For this review, take the finished solid that the model builds, in its own axes (mm). Give positions to 0.01 mm unless a question says otherwise; leave off trailing zeros. Order: outer loops, then holes, each group sorted by start corner. A loop starts at its lowest first (then second) coordinate and runs counter-clockwise, first axis right, second up.
Autodesk Inventor part; units mm, degrees
ref_plane "YZ Plane" through (0, 0, 0) normal (1, 0, 0) x (0, 1, 0)
ref_plane "XZ Plane" through (0, 0, 0) normal (0, 1, 0) x (-1, 0, 0)
ref_plane "XY Plane" through (0, 0, 0) normal (0, 0, 1) x (1, 0, 0)
ref_plane "Work Plane1" through (0, 0, 0) normal (0, 0, 1) x (1, 0, 0)
sketch "Sketch1" plane through (0, 0, 0) normal (0, 0, 1) x (1, 0, 0)
  line L0 (60, 154.3122) -> (60, -124.8582) construction
  line L1 (-40, -55.6878) -> (-40, 204.3122)
  line L2 (-40, 204.3122) -> (160, 204.3122)
  line L3 (160, 204.3122) -> (160, -55.6878)
  arc A0 (-2.8578, 10.3642) -> (-5.2959, -9.3561) centre (-2.949, 0.3646) ccw
  arc A1 (20.3319, 92.7038) -> (13.1645, 74.1711) centre (17.8081, 83.0275) ccw
  arc A2 (68.5267, 149.0877) -> (51.4733, 149.0877) centre (60, 154.3122) ccw
  arc A3 (106.8355, 74.1711) -> (99.6681, 92.7038) centre (102.1919, 83.0275) ccw
  arc A4 (125.2959, -9.3561) -> (122.8578, 10.3642) centre (122.949, 0.3646) ccw
  line L4 (-3, -12.2723) -> (-3, -52.6878)
  line L5 (0.0792, 12.6334) -> (14.681, 70.7835)
  line L6 (23.7332, 94.1894) -> (51.5594, 146.1031)
  line L7 (68.4406, 146.1031) -> (96.2668, 94.1894)
  line L8 (105.319, 70.7835) -> (119.9208, 12.6334)
  line L9 (123, -12.2723) -> (123, -52.6878)
  line L10 (160, -55.6878) -> (126, -55.6878)
  line L11 (-6, -55.6878) -> (-40, -55.6878)
  line L12 (-3, -0.4636) -> (-3, -80.75)
  line L13 (17.557, 82.2366) -> (-2.7968, 1.1803)
  line L14 (54.0507, 150.7511) -> (18.1545, 83.7816)
  line L15 (101.8455, 83.7816) -> (65.9493, 150.7511)
  line L16 (122.7968, 1.1803) -> (102.443, 82.2366)
  line L17 (123, -80.75) -> (123, -0.4636)
  arc A5 (-2.7968, 1.1803) -> (-3, -0.4636) centre (3.75, -0.4636) ccw
  arc A6 (18.1545, 83.7816) -> (17.557, 82.2366) centre (24.1037, 80.5927) ccw
  arc A7 (65.9493, 150.7511) -> (54.0507, 150.7511) centre (60, 147.5622) ccw
  arc A8 (102.443, 82.2366) -> (101.8455, 83.7816) centre (95.8963, 80.5927) ccw
  arc A9 (123, -0.4636) -> (122.7968, 1.1803) centre (116.25, -0.4636) ccw
  line L18 (60, 147.5622) -> (60, 430.3186) construction
  arc A10 (-6, -55.6878) -> (-3, -52.6878) centre (-6, -52.6878) ccw
  arc A11 (-3, -12.2723) -> (-5.2959, -9.3561) centre (-6, -12.2723) ccw
  arc A12 (-2.8578, 10.3642) -> (0.0792, 12.6334) centre (-2.8305, 13.3641) ccw
  arc A13 (14.681, 70.7835) -> (13.1645, 74.1711) centre (11.7714, 71.5142) ccw
  arc A14 (20.3319, 92.7038) -> (23.7332, 94.1894) centre (21.089, 95.6067) ccw
  arc A15 (51.5594, 146.1031) -> (51.4733, 149.0877) centre (48.9153, 147.5204) ccw
  arc A16 (68.5267, 149.0877) -> (68.4406, 146.1031) centre (71.0847, 147.5204) ccw
  arc A17 (96.2668, 94.1894) -> (99.6681, 92.7038) centre (98.911, 95.6067) ccw
  arc A18 (106.8355, 74.1711) -> (105.319, 70.7835) centre (108.2286, 71.5142) ccw
  arc A19 (119.9208, 12.6334) -> (122.8578, 10.3642) centre (122.8305, 13.3641) ccw
  arc A20 (125.2959, -9.3561) -> (123, -12.2723) centre (126, -12.2723) ccw
  arc A21 (123, -52.6878) -> (126, -55.6878) centre (126, -52.6878) ccw
  point P0 (0, 0)
  point P1 (-0.563, 10.0758)
  point P2 (-3, -9.6353)
  point P3 (22.4874, 91.8652)
  point P4 (15.3233, 73.3412)
  point P5 (67.5532, 147.7587)
  point P6 (52.4468, 147.7587)
  point P7 (104.6767, 73.3412)
  point P8 (97.5126, 91.8652)
  point P9 (123, -9.6353)
  point P10 (120.563, 10.0758)
  point P11 (97.5126, 91.8652)
  point P12 (123, -55.6878)
  point P13 (123, -55.6878)
  point P14 (-3, -55.6878)
  dimension "d0" = 200
  dimension "d1" = 100
  dimension "d2" = 260
  dimension "d3" = 50
  dimension "d4" = 10
  dimension "d5" = 10
  dimension "d6" = 10
  dimension "d7" = 10
  dimension "d8" = 10
  dimension "d9" = 3
extrude "Plate1" add sketch "Sketch1" along normal blind 3 contours L1 L2 L3 L10 A21 L9 A20 A4 A19 L8 A18 A3 A17 L7 A16 A2 A15 L6 A14 A1 A13 L5 A12 A0 A11 L4 A10 L11
equation "\"d1\" = 0.5 * d0"
equation "\"d5\" = d4"
equation "\"d6\" = d4"
equation "\"d7\" = d4"
equation "\"d8\" = d4"
equation "\"d10\" = Thickness"
equation "\"BendRadius\" = Thickness"
equation "\"BendReliefWidth\" = Thickness"
equation "\"BendReliefDepth\" = 0.5 * Thickness"
equation "\"CornerReliefSize\" = 4 * Thickness"
equation "\"MinimumRemnant\" = 2 * Thickness"
equation "\"TransitionRadius\" = BendRadius"
equation "\"JacobiRadiusSize\" = BendRadius"
equation "\"GapSize\" = Thickness"
properties part number "svejselære 1"
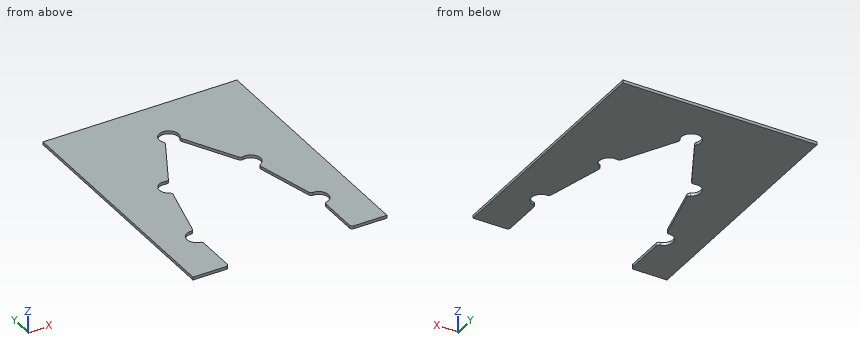
1) We need section A-A on y = 30. Give the boundary of the cut face in (x, z).
Answer sheet:
outline: (-40, 0) - (4.44, 0) - (4.44, 3) - (-40, 3) - close; (115.56, 0) - (160, 0) - (160, 3) - (115.56, 3) - close
2) Clearance check with a flat-ended pin moving along its axis: pin 1 (6 mm diameter, centred on x = -7, y = 77.5, fed in from -Z). State where the tip first meets the part, or that it passes through.
Answer sheet:
pin 1: stops at z = 0
3) We need section B-B on z = 0.5. Give the boundary of the cut face in (x, y), then the cut area to 3 significant figures.
Answer sheet:
outline: (-40, -55.69) - (-6, -55.69) arc R3 ccw to (-3, -52.69) - (-3, -12.27) arc R3 ccw to (-5.3, -9.36) arc R10 cw to (-2.86, 10.36) arc R3 ccw to (0.08, 12.63) - (14.68, 70.78) arc R3 ccw to (13.16, 74.17) arc R10 cw to (20.33, 92.7) arc R3 ccw to (23.73, 94.19) - (51.56, 146.1) arc R3 ccw to (51.47, 149.09) arc R10 cw (long way) to (68.53, 149.09) arc R3 ccw to (68.44, 146.1) - (96.27, 94.19) arc R3 ccw to (99.67, 92.7) arc R10 cw to (106.84, 74.17) arc R3 ccw to (105.32, 70.78) - (119.92, 12.63) arc R3 ccw to (122.86, 10.36) arc R10 cw to (125.3, -9.36) arc R3 ccw to (123, -12.27) - (123, -52.69) arc R3 ccw to (126, -55.69) - (160, -55.69) - (160, 204.31) - (-40, 204.31) - close
area: 32,000 mm2
4) We need section D-D on x = 32. Give the boundary of the cut face in (y, z), then the cut area to 3 significant figures.
Answer sheet:
outline: (109.61, 0) - (204.31, 0) - (204.31, 3) - (109.61, 3) - close
area: 284 mm2
5) We need section C-C on x = 60. Give the boundary of the cut face in (y, z).
Answer sheet:
outline: (164.31, 0) - (204.31, 0) - (204.31, 3) - (164.31, 3) - close
6) To check wall thickness, follow line 1 (X direction, y = -29, z = 1.4); line 2 (X direction, y = 107, z = 1.15); line 3 (Y direction, x = 102.5, z = 0.5). State the ranges of each line that lie inside material, in increasing order.
Answer sheet:
line 1: x = -40 to -3, 123 to 160
line 2: x = -40 to 30.6, 89.4 to 160
line 3: y = 93.02 to 204.31
